CAD build for the part. Positions are in the model's coordinates, mm. A direction names the side the tool comes from. Coordinates: 2 decimals unless noted, no trailing zeros. Loops run counter-clockwise (first coordinate to the right, second up) from the corner with the lowest first, then second, coordinate; pieces in that order, holes last. Notation, with made-up numbers: (-36, -6.75) -> (-17, -6.75) arc R32 cw to (-17, 31.25) -> close; hole circle Ø6 at (32, -33). An arc over 180 degrees is marked (long way). Return JSON: item names as keys, results as strings. Group by question number.
(1) Saw through at B-B on y = 45. Write the cut outline in (x, z), then the cut area to 3 significant figures.
(2) Saw through at A-A on x = 30. Write the cut outline in (y, z), then the cut area to 3 significant figures.
(3) Probe L1, parallel to Y at x = 5, z = 1.15; L2, parallel to Y at x = 17.5, z = 68.2; L3, parallel to X at y = 11, z = 23. List the from-to ranges inside material, lowest first.
(4) Mould opens along Z. For faces 5 (the face through (3.25, 30.08, 2.46)), 6 (the face through (17.4, 32.6, 67)), 7 (the face through (44, 18, 80)) say: pulls with the +Z half, pulls with the -Z half, needs draft (parallel to the pull), parting line crosses it, or undercut.
(5) Saw through at C-C on y = 5. Write the cut outline in (x, z), then the cut area to 3 significant figures.
(6) Flat gauge pins, fed straight in: pin 1 Ø12 at (x, y) = (41, 24) entering from +Z; pin 2 Ø6 at (x, y) = (17.5, 35) entering from +Z; pin 3 Ø4.5 at (x, y) = (81.5, 5) entering from -Z; pin 4 Ø5.5 at (x, y) = (5, 30) entering from -Z. Where does each tip first touch, or does it go through?
(7) Tool access for faces 1 (the face through (10, 17, 30)), 2 (the face through (25, 18, 40)), 3 (the face through (0, 17, 2)), 4 (the face through (-3, 18, 57)): list every direction of +Z, -Z, +X, -X, +Y, -Y with a clear straight run to the whole face (end or side of a thin tool).
(8) Saw through at D-D on x = -10. Write the cut outline in (y, z).
```python
from build123d import *

# Parameters (mm, degrees)
SKETCH_W     = 35
SKETCH_H     = 35
SKETCH_R     = 1.75
PAD_DEPTH    = 5
SKETCH001_W  = 15
SKETCH001_H  = 15
PAD001_DEPTH = 50
SKETCH002_W  = 40
SKETCH002_H  = 15
SKETCH002_R  = 2.25
PAD002_DEPTH = 2
SKETCH003_W  = 15
SKETCH003_H  = 15
PAD003_DEPTH = 10
SKETCH004_W  = 15
SKETCH004_H  = 30
SKETCH004_R  = 2.25
PAD004_DEPTH = 2
SKETCH005_W  = 15
SKETCH005_H  = 15
PAD005_DEPTH = 6
SKETCH006_R  = 2.25
PAD006_DEPTH = 5
SKETCH007_W  = 15
SKETCH007_H  = 30
SKETCH007_R  = 2.25
PAD007_DEPTH = 2
SKETCH008_W  = 25
SKETCH008_H  = 3
POCKET_DEPTH = 25


with BuildPart() as part:
    # Sketch → Pad (new body)
    with BuildSketch(Plane.XY):
        with Locations((17.5, 17.5)):
            Rectangle(SKETCH_W, SKETCH_H)
        with Locations((5, 5)):
            Circle(SKETCH_R, mode=Mode.SUBTRACT)
        with Locations((5, 30)):
            Circle(SKETCH_R, mode=Mode.SUBTRACT)
        with Locations((30, 30)):
            Circle(SKETCH_R, mode=Mode.SUBTRACT)
        with Locations((30, 5)):
            Circle(SKETCH_R, mode=Mode.SUBTRACT)
    extrude(amount=PAD_DEPTH)

    # Sketch001 (on Face10 of Pad) → Pad001 (join)
    with BuildSketch(Plane.XY.offset(5)):
        with Locations((17.5, 17.5)):
            Rectangle(SKETCH001_W, SKETCH001_H)
    extrude(amount=PAD001_DEPTH)

    # Sketch002 (on Face15 of Pad001) → Pad002 (join)
    with BuildSketch(Plane.XY.offset(55)):
        with Locations((5, 17.5)):
            Rectangle(SKETCH002_W, SKETCH002_H)
        with Locations((-10, 17.5)):
            Circle(SKETCH002_R, mode=Mode.SUBTRACT)
    extrude(amount=PAD002_DEPTH)

    # Sketch003 (on Face21 of Pad002) → Pad003 (join)
    with BuildSketch(Plane.XY.offset(57)):
        with Locations((17.5, 17.5)):
            Rectangle(SKETCH003_W, SKETCH003_H)
    extrude(amount=PAD003_DEPTH)

    # Sketch004 (on Face26 of Pad003) → Pad004 (join)
    with BuildSketch(Plane.XY.offset(67)):
        with Locations((17.5, 25)):
            Rectangle(SKETCH004_W, SKETCH004_H)
        with Locations((17.5, 35)):
            Circle(SKETCH004_R, mode=Mode.SUBTRACT)
    extrude(amount=PAD004_DEPTH)

    # Sketch005 (on Face30 of Pad004) → Pad005 (join)
    with BuildSketch(Plane.XY.offset(69)):
        with Locations((17.5, 17.5)):
            Rectangle(SKETCH005_W, SKETCH005_H)
    extrude(amount=PAD005_DEPTH)

    # Sketch006 (on Face36 of Pad005) → Pad006 (join)
    with BuildSketch(Plane.XY.offset(75)):
        Polygon((10, 25), (77.5, 25), (77.5, 50), (92.5, 50), (92.5, 10), (10, 10), align=None)
        with Locations((85, 45)):
            Circle(SKETCH006_R, mode=Mode.SUBTRACT)
    extrude(amount=PAD006_DEPTH)

    # Sketch007 (on Face41 of Pad006) → Pad007 (join)
    with BuildSketch(Plane.XY.offset(80)):
        with Locations((85, 10)):
            Rectangle(SKETCH007_W, SKETCH007_H)
        with Locations((85, 0)):
            Circle(SKETCH007_R, mode=Mode.SUBTRACT)
    extrude(amount=PAD007_DEPTH)

    # Sketch008 (on Face40 of Pad007) → Pocket (cut)
    with BuildSketch(Plane.YZ.offset(92.5)):
        with Locations((37.5, 78.5)):
            Rectangle(SKETCH008_W, SKETCH008_H)
    extrude(amount=-POCKET_DEPTH, mode=Mode.SUBTRACT)


solid = part.part
```
Geometry results:
{
 "1": {"outline": "(77.5, 75) -> (82.75, 75) -> (82.75, 77) -> (77.5, 77) -> close; (87.25, 75) -> (92.5, 75) -> (92.5, 77) -> (87.25, 77) -> close", "area": "21.0 mm²"},
 "2": {"outline": "(0, 0) -> (3.25, 0) -> (3.25, 5) -> (0, 5) -> close; (6.75, 0) -> (28.25, 0) -> (28.25, 5) -> (6.75, 5) -> close; (10, 75) -> (25, 75) -> (25, 80) -> (10, 80) -> close; (31.75, 0) -> (35, 0) -> (35, 5) -> (31.75, 5) -> close", "area": "215 mm²"},
 "3": {"L1": "0 to 3.25, 6.75 to 28.25, 31.75 to 35", "L2": "10 to 32.75, 37.25 to 40", "L3": "10 to 25"},
 "4": {"face 5": "needs draft", "face 6": "undercut", "face 7": "pulls with the +Z half"},
 "5": {"outline": "(0, 0) -> (3.25, 0) -> (3.25, 5) -> (0, 5) -> close; (6.75, 0) -> (28.25, 0) -> (28.25, 5) -> (6.75, 5) -> close; (31.75, 0) -> (35, 0) -> (35, 5) -> (31.75, 5) -> close; (77.5, 80) -> (92.5, 80) -> (92.5, 82) -> (77.5, 82) -> close", "area": "170 mm²"},
 "6": {"pin 1": "z = 80", "pin 2": "z = 69", "pin 3": "z = 80", "pin 4": "z = 0"},
 "7": {"face 1": "-X, +Y, -Y", "face 2": "+X, +Y, -Y", "face 3": "-Z, -X, +Y, -Y", "face 4": "+Z, -X, +Y, -Y"},
 "8": {"outline": "(10, 55) -> (15.25, 55) -> (15.25, 57) -> (10, 57) -> close; (19.75, 55) -> (25, 55) -> (25, 57) -> (19.75, 57) -> close"}
}
